```python
from build123d import *

# Parameters (mm, degrees)
RESSALTO_EXTRUS_O1_DEPTH = 3.5
ESBO_O15_W               = 33
ESBO_O15_H               = 14
ESBO_O15_R               = 2
ESBO_O15_H_2             = 7
RESSALTO_EXTRUS_O2_DEPTH = 3
ESBO_O16_R               = 1.75
CORTE_EXTRUS_O1_DEPTH    = 58.554322166


with BuildPart() as part:
    # Esboço14 → Ressalto-extrusão1 (new, symmetric)
    with BuildSketch(Plane(origin=(0, 0, 0), x_dir=(1, 0, 0), z_dir=(0, 1, 0))):
        Polygon((-12, 2.5), (-17, 2.5), (-17, 20), (-50, 20), (-50, 17), (-24, 17), (-24, -2.5), (-12, -2.5), align=None)
    extrude(amount=RESSALTO_EXTRUS_O1_DEPTH, both=True)

    # Esboço15 → Ressalto-extrusão2 (add)
    with BuildSketch(Plane(origin=(0, 0, -20), x_dir=(-1, 0, 0), z_dir=(0, 0, -1))):
        with Locations((33.5, -10.5)):
            Rectangle(ESBO_O15_W, ESBO_O15_H)
        with Locations((21, -12.75)):
            Circle(ESBO_O15_R, mode=Mode.SUBTRACT)
        with Locations((46, -12.75)):
            Circle(ESBO_O15_R, mode=Mode.SUBTRACT)
        with Locations((33.5, 10.5)):
            Rectangle(ESBO_O15_W, ESBO_O15_H)
        with Locations((21, 12.75)):
            Circle(ESBO_O15_R, mode=Mode.SUBTRACT)
        with Locations((46, 12.75)):
            Circle(ESBO_O15_R, mode=Mode.SUBTRACT)
        with Locations((33.5, 0)):
            Rectangle(ESBO_O15_W, ESBO_O15_H_2)
    extrude(amount=-RESSALTO_EXTRUS_O2_DEPTH)

    # Esboço16 → Corte-extrusão1 (cut, through all)
    with BuildSketch(Plane.XY.offset(2.5)):
        with Locations((-21, 0)):
            Circle(ESBO_O16_R)
    extrude(amount=-CORTE_EXTRUS_O1_DEPTH, mode=Mode.SUBTRACT)

    # Varredura1: sweep along a path in Esboço1
    with BuildLine(Plane.XY) as varredura1_path:
        ThreePointArc((7.070663707, 8.426488874), (-11, 0), (7.070663707, -8.426488874))
    # 3DSketch2 → Varredura1 (sweep)
    with BuildSketch(Plane(origin=(8.034845121, -9.575555539, 2.5), x_dir=(-0.33071149682512846, 0.39412661445355873, -0.8574929257125443), z_dir=(0.7660444431189768, 0.6427876096865409, 3.624573608241852e-15))):
        Polygon((0, 0), (1.543487266, 2.572478777), (5.830951895, 0), (4.287464629, -2.572478777), align=None)
    sweep(path=varredura1_path.line)


solid = part.part
```
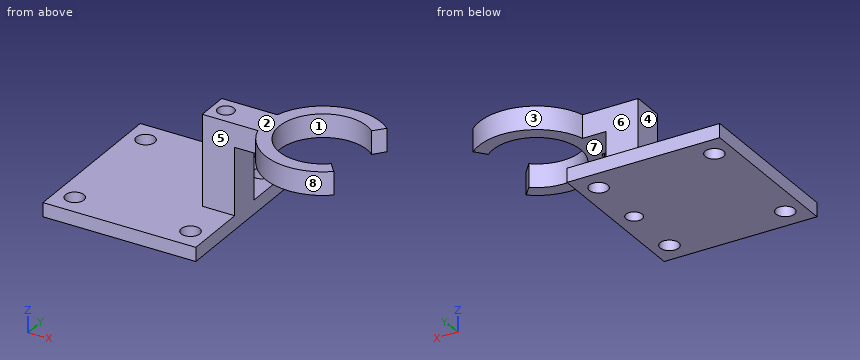
Geometry check sheet. Reference: the model listing, model coordinates, mm. Face numbers are marked on the shaded views. A direction names the side the tool comes from. Coordinates: 2 decimals unless noted, no trailing zeros. Order: outer loops, then holes, each group sorted by start corner. A loop starts at its lowest first (then second) coordinate and runs counter-clockwise, first axis right, second up.
Item 1: Section check B-B (y = 0). Enter the section's corners in (x, z), plus the area to 3 significant figures.
Item 2: Tool access check on the marked faces 4, 5, 6, 7 and 8. Record the directions out of +Z, -Z, +X, -X, +Y, -Y that give a thin tool (end or side, any length) a straight path to the whole face; none if there is none.
Item 3: Section check D-D (z = -9.75). Enter the section's corners in (x, y), plus the area to 3 significant figures.
Item 4: Section check A-A (x = -21). Enter the section's corners in (y, z), plus the area to 3 significant figures.
Item 5: Scan lines: line 1 along Y through (x, z) = (-46, -17.8); line 2 along Y through (x, z) = (-21, -3.5); line 3 along Z through (x, y) = (-45, -5.5). Record each from-to range of solid material in increasing order.
Item 6: Section check C-C (x = -46). Enter the section's corners in (y, z), plus the area to 3 significant figures.
Item 7: Depth check by flat-ended pin: pin 1 (12.5 mm diameter, centred on x = -5.5, y = -1.5, fed in from -Z); pin 2 (5 mm diameter, centred on x = -40, y = 6, fed in from +Z); pin 3 (5.5 mm diameter, centred on y = 1.5, z = -10, fed in from -X); pin 4 (4 mm diameter, centred on y = -6, z = -15.5, fed in from -X). Enter the tip coordinate at first touch or a pass-through.
Item 8: Mould release check, pull along X, two halves, no side actions. Record for the marked faces 1, 2 and 3: released by +X, released by -X, zero draft, split by the parting line, or undercut.
Check sheet entries:
1. outline: (-50, -20) - (-22.75, -20) - (-22.75, 2.5) - (-24, 2.5) - (-24, -17) - (-50, -17) - close; (-19.25, -20) - (-17, -20) - (-17, -2.5) - (-9.5, -2.5) - (-9.5, 2.5) - (-19.25, 2.5) - close
1. area: 194 mm2
2. face 4: +Z, -X, +Y, -Y
2. face 5: +Z, -X, -Y
2. face 6: +Z, -X, +Y
2. face 7: -Z, +X, +Y, -Y
2. face 8: +Z, -Z, -Y
3. outline: (-24, -3.5) - (-17, -3.5) - (-17, 3.5) - (-24, 3.5) - close; hole circle Ø3.5 at (-21, 0)
3. area: 39.4 mm2
4. outline: (-17.5, -20) - (-14.75, -20) - (-14.75, -17) - (-17.5, -17) - close; (-10.75, -20) - (-1.75, -20) - (-1.75, 2.5) - (-3.5, 2.5) - (-3.5, -17) - (-10.75, -17) - close; (1.75, -20) - (10.75, -20) - (10.75, -17) - (3.5, -17) - (3.5, 2.5) - (1.75, 2.5) - close; (14.75, -20) - (17.5, -20) - (17.5, -17) - (14.75, -17) - close
4. area: 139 mm2
5. line 1: y = -17.5 to -14.75, -10.75 to 10.75, 14.75 to 17.5
5. line 2: y = -3.5 to -1.75, 1.75 to 3.5
5. line 3: z = -20 to -17
6. outline: (-17.5, -20) - (-14.75, -20) - (-14.75, -17) - (-17.5, -17) - close; (-10.75, -20) - (10.75, -20) - (10.75, -17) - (-10.75, -17) - close; (14.75, -20) - (17.5, -20) - (17.5, -17) - (14.75, -17) - close
6. area: 81.0 mm2
7. pin 1: stops at z = -2.5
7. pin 2: stops at z = -17
7. pin 3: stops at x = -24
7. pin 4: stops at x = -50
8. face 1: undercut
8. face 2: zero draft
8. face 3: split by the parting line
